For this review, use the dimensioned drawing (mm, ordinates from the lowest corner) and the shaded views. Give positions to 0.01 mm unless a question says otherwise; leave off trailing zeros. Write each loop counter-clockwise with the first axis right and the second up, starting at its lowest first coordinate (ties: lowest second). Pieces come first, ordered by that corner, then holes. Notation, with made-up numbers: (-19.5, 54.25) -> (30.5, 54.25) arc R37 cw to (30.5, 91.25) -> close; hole circle Ø1 at (4, 30.25). An arc over 180 degrees is marked (long way). Return JSON: item names as keys, results as strings.
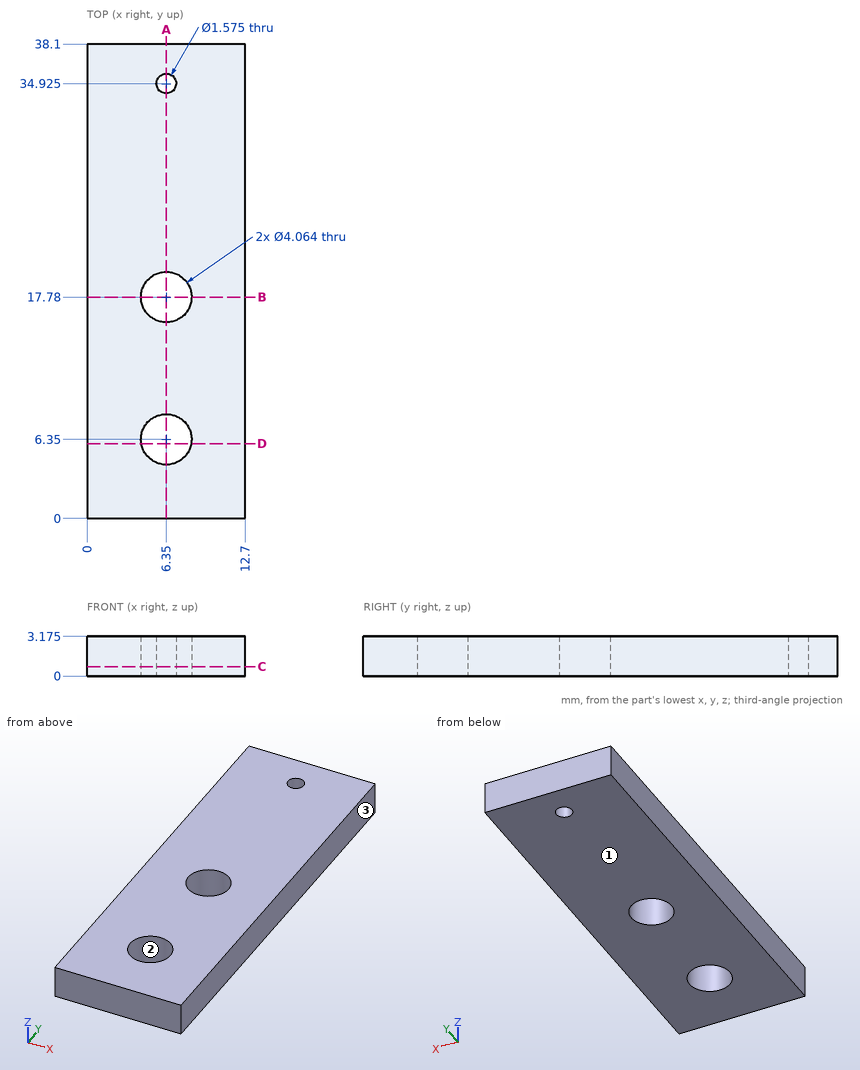
1. Add section B-B, the plane y = 17.78. State the section outline as (x, z) points (3 decimals), plus the area to 3 significant figures.
Results found:
{"outline": "(0, 0) -> (4.318, 0) -> (4.318, 3.175) -> (0, 3.175) -> close; (8.382, 0) -> (12.7, 0) -> (12.7, 3.175) -> (8.382, 3.175) -> close", "area": "27.4 mm²"}
2. The part is to be moulded in two halves that separate along X. For the marked faces 1, 2 and 3, say which applies: +X half, -X half, draft (parallel to the pull), parting line (faces both ways), or undercut.
Results found:
{"face 1": "draft", "face 2": "undercut", "face 3": "+X half"}
3. To check wall thickness, follow probe 1 along Y at (x, z) = (6.35, 1.8); probe 2 along X at (y, z) = (6.35, 2); probe 3 along Y at (x, z) = (8, 2.3) (1 decimal). State the ranges of each line that lie inside material, in increasing order.
Results found:
{"probe 1": "y = 0 to 4.32, 8.38 to 15.75, 19.81 to 34.14, 35.71 to 38.1", "probe 2": "x = 0 to 4.32, 8.38 to 12.7", "probe 3": "y = 0 to 5.2, 7.5 to 16.6, 19 to 38.1"}
4. Add section C-C, the plane z = 0.75. Count the separate pieces of the cut face and the enclosed holes in it, plus the area to 3 significant figures.
Results found:
{"separate pieces": "1", "enclosed holes": "3", "area": "456 mm²"}
5. Add section A-A, the plane x = 6.35. State the section outline as (y, z) points (1 decimal).
Results found:
{"outline": "(0, 0) -> (4.3, 0) -> (4.3, 3.2) -> (0, 3.2) -> close; (8.4, 0) -> (15.7, 0) -> (15.7, 3.2) -> (8.4, 3.2) -> close; (19.8, 0) -> (34.1, 0) -> (34.1, 3.2) -> (19.8, 3.2) -> close; (35.7, 0) -> (38.1, 0) -> (38.1, 3.2) -> (35.7, 3.2) -> close"}
6. Add section D-D, the plane y = 6. State the section outline as (x, z) points (1 decimal), plus the area to 3 significant figures.
Results found:
{"outline": "(0, 0) -> (4.3, 0) -> (4.3, 3.2) -> (0, 3.2) -> close; (8.4, 0) -> (12.7, 0) -> (12.7, 3.2) -> (8.4, 3.2) -> close", "area": "27.6 mm²"}
